Input: part model. Units: mm. Frame: model coordinates. Face numbers are marked on the shaded views. A direction names the side the tool comes from. Coordinates: 2 decimals unless noted, no trailing zeros. Order: outer loops, then holes, each group sorted by start corner. A loop starts at its lowest first (then second) coordinate and runs counter-clockwise, first axis right, second up. Notation, with made-up numbers: M -20,-4 L -14,-4 A20 ccw -14,2 Z; hole C 81.5,40 d2. An arc over 180 degrees is marked long. One line per item, written item: value.
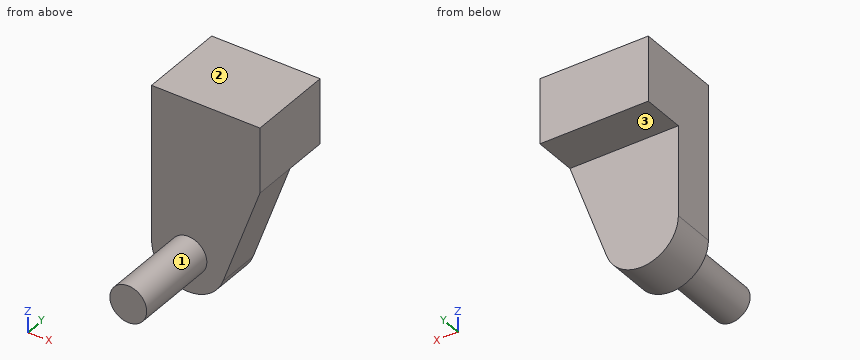
```python
from build123d import *

# Parameters (mm, degrees)
F0_W     = 63.5
F0_H     = 38.1
F1_DEPTH = 25.4
F2_R     = 10.795746
F3_DEPTH = 76.2
F4_W     = 63.5
F4_H     = 38.1
F5_DEPTH = 25.4


with BuildPart() as f1:
    # F0 (on Front) → F1 (new body)
    with BuildSketch(Plane.XZ):
        with Locations((-2.008985, 33.25243)):
            Rectangle(F0_W, F0_H)
        with BuildLine():
            Line((29.741015, 14.20243), (-33.758985, 14.20243))
            Line((-33.758985, 14.20243), (-33.758985, -38.45109))
            ThreePointArc((-33.758985, -38.45109), (-12.168985, -16.86109), (9.421015, -38.45109))
            ThreePointArc((9.421015, -38.45109), (9.099334, -42.164136), (8.143877, -45.766536))
            Line((8.143877, -45.766536), (29.741015, 14.20243))
        make_face()
        with BuildLine():
            ThreePointArc((9.421015, -38.45109), (-12.168985, -16.86109), (-33.758985, -38.45109))
            ThreePointArc((-33.758985, -38.45109), (-15.88203, -59.71941), (8.143877, -45.766536))
            ThreePointArc((8.143877, -45.766536), (9.099334, -42.164136), (9.421015, -38.45109))
        make_face()
    extrude(amount=F1_DEPTH)

    # F2 (on Front) → F3 (join)
    with BuildSketch(Plane.XZ):
        with Locations((-12.168985, -38.45109)):
            Circle(F2_R)
    extrude(amount=F3_DEPTH)

    # F4 (on face) → F5 (join)
    with BuildSketch(Plane(origin=(0, 0, 0), x_dir=(-1, 0, 0), z_dir=(0, 1, 0))):
        with Locations((2.008985, 33.25243)):
            Rectangle(F4_W, F4_H)
    extrude(amount=F5_DEPTH)


solid = f1.part
```
(1) Cut plane B-B on x = -7.5. Output: boundary loops of the cut face in (y, z), plus the area to 3 significant figures.
Data:
outline: M -76.2,-48.18 L -25.4,-48.18 L -25.4,-59.53 L 0,-59.53 L 0,14.2 L 25.4,14.2 L 25.4,52.3 L -25.4,52.3 L -25.4,-28.72 L -76.2,-28.72 Z
area: 4,800 mm2
(2) Ray query, line 1 (Y direction, x = 14.5, z = 10); line 2 (Y direction, x = -6.5, z = 32.5); line 3 (Z direction, x = -9.5, y = 19.5). Return the intervals inside material, ascending. Write a range as from..to.
Data:
line 1: y = -25.4..0
line 2: y = -25.4..25.4
line 3: z = 14.2..52.3
(3) Cut plane C-C on y = 17.5. Output: boundary loops of the cut face in (x, z).
Data:
outline: M -33.76,14.2 L 29.74,14.2 L 29.74,52.3 L -33.76,52.3 Z
(4) Access query for the marked faces 1, 2 and 3. Directions: +Z, -Z, +X, -X, +Y, -Y. A direction counts if a zero-diameter tool reaches every point of the face in a straight line with its end or side. Return the directions, or none.
Data:
face 1: -Y
face 2: +Z, +X, -X, +Y, -Y
face 3: -Z, +X, -X, +Y
(5) Cut plane D-D on x = 17. Output: boundary loops of the cut face in (y, z).
Data:
outline: M -25.4,-21.18 L 0,-21.18 L 0,14.2 L 25.4,14.2 L 25.4,52.3 L -25.4,52.3 Z
(6) First-contact query: pin 1 (5 mm diameter, centred on x = -12.5, y = -60.5, fed in from -Z); pin 2 (6 mm diameter, centred on x = 3, y = -11, fed in from -Z); pin 3 (6 mm diameter, centred on x = -13.5, z = 1, fed in from -Y). Flat tips, straight axial feed; report the tip coordinate or a pass-through.
Data:
pin 1: stops at z = -49.25
pin 2: stops at z = -56.28
pin 3: stops at y = -25.4
(7) Cut plane A-A on z = -33. Output: boundary loops of the cut face in (x, y), plus the area to 3 significant figures.
Data:
outline: M -33.76,-25.4 L -21.49,-25.4 L -21.49,-76.2 L -2.85,-76.2 L -2.85,-25.4 L 12.74,-25.4 L 12.74,0 L -33.76,0 Z
area: 2,130 mm2
